Work out the finished part from the listing and answer in its coordinate system (mm). A direction names the side the tool comes from. Coordinates: 2 decimals unless noted, no trailing zeros. Order: outer loops, then holes, each group sorted by start corner. A loop starts at its lowest first (then second) coordinate and runs counter-clockwise, first axis right, second up. Notation, with made-up numbers: (69, 63.5) -> (105, 63.5) arc R5 cw to (105, 72.5) -> close; hole circle Ø10 at (59, 84.25). An arc over 180 degrees is marked (long way). Write item = value, one per line. Start each with the question number.
Q1. Straight lines are drawn through the part: L1, parallel to Z at x = 156, y = 10.5; L2, parallel to Z at x = 177, y = 2; L3, parallel to Y at x = 27.5, z = -49. For each, find the intervals that lie inside material, in ascending order. Write a range as from..to.
Q2. The part is cut by section B-B, the plane y = 13.5. Determine the outline of the cut face in (x, z), plus the area to 3 significant figures.
Q3. For a pull along X with two mould halves and no side action, classify faces 3 (the cylindrical face through (92.904, 1.521, -22.261)), 4 (the flat face through (-3, 0, -26)) as +X half, -X half, draft (parallel to the pull), parting line (faces both ways), or undercut.
Q4. The part is cut by section A-A, the plane x = -100. Determine the outline of the cut face in (y, z).
Q5. Flat-ended cylindrical pins translate along their axes: pin 1 (10.5 mm diameter, centred on x = 48.79, z = -48.79, fed in from +Y); pin 2 (4.5 mm diameter, centred on y = 10, z = -57, fed in from -X); pin 3 (0.9 mm diameter, centred on x = 175, y = 1, fed in from -Z). Find the tip coordinate at first contact, or state that the pin passes through.
Q6. Which of the six approach directions +Z, -Z, +X, -X, +Y, -Y give full straight-line access (tool end or side, diameter ignored) to faces 1 (the cylindrical face through (107.096, 1.521, 22.261)), 2 (the flat face through (2, 15, -57))?
Q7. The part is cut by section C-C, the plane x = 135. Determine the outline of the cut face in (y, z), plus the area to 3 significant figures.
```python
from build123d import *

# Parameters (mm, degrees)
SKETCH1_W                      = 370
SKETCH1_H                      = 114
SKETCH1_R                      = 4
SKETCH1_R_2                    = 24.5
BOSS_EXTRUDE1_DEPTH            = 3
EDGE_FLANGE1_STRIP_W           = 14
EDGE_FLANGE1_STRIP_H           = 3
EDGE_FLANGE1_STRIP_CUT_DEPTH   = 370
EDGE_FLANGE1_STRIP_2_W         = 14
EDGE_FLANGE1_STRIP_2_H         = 3
EDGE_FLANGE1_STRIP_CUT_2_DEPTH = 370
EDGE_FLANGE1_DEPTH             = 370
EDGE_FLANGE1_BEND_DEPTH        = 370
CUT_EXTRUDE1_REACH             = 198.087
SKETCH16_R                     = 3
SKETCH16_W                     = 25
SKETCH16_H                     = 58
CUT_EXTRUDE2_REACH             = 197.727
SKETCH17_R                     = 10.5
CUT_EXTRUDE3_START             = -185
CUT_EXTRUDE3_DEPTH             = 28
CUT_EXTRUDE3_START_2           = 157
CUT_EXTRUDE3_2_DEPTH           = 28


# Read off the part's stored shape, not the designer's step: Cut-Extrude3
# Sheet-metal steps are written as plain solids
with BuildPart() as part:
    # Sketch1 → Boss-Extrude1 (new body)
    with BuildSketch(Plane(origin=(0, 0, 0), x_dir=(1, 0, 0), z_dir=(0, 1, 0))):
        Rectangle(SKETCH1_W, SKETCH1_H)
        with Locations(Location((-48.790367902, 48.790367902, 0), (0, 0, 270))):
            Circle(SKETCH1_R, mode=Mode.SUBTRACT)
        with Locations(Location((48.790367902, 48.790367902, 0), (0, 0, 270))):
            Circle(SKETCH1_R, mode=Mode.SUBTRACT)
        with Locations(Location((48.790367902, -48.790367902, 0), (0, 0, 270))):
            Circle(SKETCH1_R, mode=Mode.SUBTRACT)
        with Locations(Location((-48.790367902, -48.790367902, 0), (0, 0, 270))):
            Circle(SKETCH1_R, mode=Mode.SUBTRACT)
        with Locations(Location((0, 0, 0), (0, 0, 270))):
            Circle(SKETCH1_R_2, mode=Mode.SUBTRACT)
    extrude(amount=BOSS_EXTRUDE1_DEPTH)

    # Edge-Flange1 strip (across the edge) → Edge-Flange1 strip cut (cut)
    with BuildSketch(Plane(origin=(-185, 3, 57), x_dir=(0, 0, -1), z_dir=(1, 0, 0))):
        with Locations((-6, -1.5)):
            Rectangle(EDGE_FLANGE1_STRIP_W, EDGE_FLANGE1_STRIP_H)
    extrude(amount=EDGE_FLANGE1_STRIP_CUT_DEPTH, mode=Mode.SUBTRACT)

    # Edge-Flange1 strip 2 (across the edge) → Edge-Flange1 strip cut 2 (cut)
    with BuildSketch(Plane(origin=(185, 3, -57), x_dir=(0, 0, 1), z_dir=(-1, 0, 0))):
        with Locations((-6, -1.5)):
            Rectangle(EDGE_FLANGE1_STRIP_2_W, EDGE_FLANGE1_STRIP_2_H)
    extrude(amount=EDGE_FLANGE1_STRIP_CUT_2_DEPTH, mode=Mode.SUBTRACT)

    # Edge-Flange1 section (across the edge) → Edge-Flange1 (add)
    with BuildSketch(Plane(origin=(-185, 3, 57), x_dir=(0, 0, -1), z_dir=(1, 0, 0))):
        with BuildLine():
            Line((-3, 1), (-3, 22))
            Line((-3, 22), (0, 22))
            Line((0, 22), (0, 1))
            ThreePointArc((0, 1), (0.292893219, 0.292893219), (1, 0))
            Line((1, 0), (1, -3))
            ThreePointArc((1, -3), (-1.828427125, -1.828427125), (-3, 1))
        make_face()
    extrude(amount=EDGE_FLANGE1_DEPTH)

    # Edge-Flange1 section 2 (across the edge) → Edge-Flange1 bend (add)
    with BuildSketch(Plane(origin=(185, 3, -57), x_dir=(0, 0, 1), z_dir=(-1, 0, 0))):
        with BuildLine():
            Line((-3, 1), (-3, 22))
            Line((-3, 22), (0, 22))
            Line((0, 22), (0, 1))
            ThreePointArc((0, 1), (0.292893219, 0.292893219), (1, 0))
            Line((1, 0), (1, -3))
            ThreePointArc((1, -3), (-1.828427125, -1.828427125), (-3, 1))
        make_face()
    extrude(amount=EDGE_FLANGE1_BEND_DEPTH)

    # Sketch16 → Cut-Extrude1 (cut, up to next)
    with BuildSketch(Plane.XZ, mode=Mode.PRIVATE) as cut_extrude1_sk1:
        with Locations(Location((177, 0, 0), (0, 0, 270))):
            Circle(SKETCH16_R)
    cut_extrude1_tool1 = extrude(cut_extrude1_sk1.sketch, amount=-CUT_EXTRUDE1_REACH, mode=Mode.PRIVATE) & part.part
    # Sketch16 → Cut-Extrude1 (cut, up to next)
    with BuildSketch(Plane.XZ, mode=Mode.PRIVATE) as cut_extrude1_sk2:
        with Locations(Location((145, 0, 0), (0, 0, 270))):
            Circle(SKETCH16_R)
    cut_extrude1_tool2 = extrude(cut_extrude1_sk2.sketch, amount=-CUT_EXTRUDE1_REACH, mode=Mode.PRIVATE) & part.part
    # Sketch16 → Cut-Extrude1 (cut, up to next)
    with BuildSketch(Plane.XZ, mode=Mode.PRIVATE) as cut_extrude1_sk3:
        with Locations((-172.5, 0)):
            Rectangle(SKETCH16_W, SKETCH16_H)
    cut_extrude1_tool3 = extrude(cut_extrude1_sk3.sketch, amount=-CUT_EXTRUDE1_REACH, mode=Mode.PRIVATE) & part.part
    add(cut_extrude1_tool1.solids().sort_by_distance((177, 0, 0))[0], mode=Mode.SUBTRACT)
    add(cut_extrude1_tool2.solids().sort_by_distance((145, 0, 0))[0], mode=Mode.SUBTRACT)
    add(cut_extrude1_tool3.solids().sort_by_distance((-172.5, 0, 0))[0], mode=Mode.SUBTRACT)

    # Sketch17 → Cut-Extrude2 (cut, up to next)
    with BuildSketch(Plane(origin=(0, 3, 0), x_dir=(1, 0, 0), z_dir=(0, 1, 0)), mode=Mode.PRIVATE) as cut_extrude2_sk1:
        with Locations(Location((-100, 30, 0), (0, 0, 270))):
            Circle(SKETCH17_R)
    cut_extrude2_tool1 = extrude(cut_extrude2_sk1.sketch, amount=-CUT_EXTRUDE2_REACH, mode=Mode.PRIVATE) & part.part
    # Sketch17 → Cut-Extrude2 (cut, up to next)
    with BuildSketch(Plane(origin=(0, 3, 0), x_dir=(1, 0, 0), z_dir=(0, 1, 0)), mode=Mode.PRIVATE) as cut_extrude2_sk2:
        with Locations(Location((100, 30, 0), (0, 0, 90))):
            Circle(SKETCH17_R)
    cut_extrude2_tool2 = extrude(cut_extrude2_sk2.sketch, amount=-CUT_EXTRUDE2_REACH, mode=Mode.PRIVATE) & part.part
    # Sketch17 → Cut-Extrude2 (cut, up to next)
    with BuildSketch(Plane(origin=(0, 3, 0), x_dir=(1, 0, 0), z_dir=(0, 1, 0)), mode=Mode.PRIVATE) as cut_extrude2_sk3:
        with Locations(Location((100, -30, 0), (0, 0, 270))):
            Circle(SKETCH17_R)
    cut_extrude2_tool3 = extrude(cut_extrude2_sk3.sketch, amount=-CUT_EXTRUDE2_REACH, mode=Mode.PRIVATE) & part.part
    # Sketch17 → Cut-Extrude2 (cut, up to next)
    with BuildSketch(Plane(origin=(0, 3, 0), x_dir=(1, 0, 0), z_dir=(0, 1, 0)), mode=Mode.PRIVATE) as cut_extrude2_sk4:
        with Locations(Location((-100, -30, 0), (0, 0, 90))):
            Circle(SKETCH17_R)
    cut_extrude2_tool4 = extrude(cut_extrude2_sk4.sketch, amount=-CUT_EXTRUDE2_REACH, mode=Mode.PRIVATE) & part.part
    add(cut_extrude2_tool1.solids().sort_by_distance((-100, 3, -30))[0], mode=Mode.SUBTRACT)
    add(cut_extrude2_tool2.solids().sort_by_distance((100, 3, -30))[0], mode=Mode.SUBTRACT)
    add(cut_extrude2_tool3.solids().sort_by_distance((100, 3, 30))[0], mode=Mode.SUBTRACT)
    add(cut_extrude2_tool4.solids().sort_by_distance((-100, 3, 30))[0], mode=Mode.SUBTRACT)

    # Cut-Extrude3 outline → Cut-Extrude3 (cut)
    with BuildSketch(Plane.YZ.offset(CUT_EXTRUDE3_START)):
        with BuildLine():
            ThreePointArc((4, -57), (3.292893219, -56.707106781), (3, -56))
            Line((3, -56), (0, -56))
            ThreePointArc((0, -56), (1.171572875, -58.828427125), (4, -60))
            Line((4, -60), (25, -60))
            Line((25, -60), (25, -57))
            Line((25, -57), (4, -57))
        make_face()
        with BuildLine():
            ThreePointArc((4, 60), (1.171572875, 58.828427125), (0, 56))
            Line((0, 56), (3, 56))
            ThreePointArc((3, 56), (3.292893219, 56.707106781), (4, 57))
            Line((4, 57), (25, 57))
            Line((25, 57), (25, 60))
            Line((25, 60), (4, 60))
        make_face()
    extrude(amount=CUT_EXTRUDE3_DEPTH, mode=Mode.SUBTRACT)

    # Cut-Extrude3 2 outline → Cut-Extrude3 2 (cut)
    with BuildSketch(Plane.YZ.offset(CUT_EXTRUDE3_START_2)):
        with BuildLine():
            ThreePointArc((4, -57), (3.292893219, -56.707106781), (3, -56))
            Line((3, -56), (0, -56))
            ThreePointArc((0, -56), (1.171572875, -58.828427125), (4, -60))
            Line((4, -60), (25, -60))
            Line((25, -60), (25, -57))
            Line((25, -57), (4, -57))
        make_face()
        with BuildLine():
            ThreePointArc((4, 60), (1.171572875, 58.828427125), (0, 56))
            Line((0, 56), (3, 56))
            ThreePointArc((3, 56), (3.292893219, 56.707106781), (4, 57))
            Line((4, 57), (25, 57))
            Line((25, 57), (25, 60))
            Line((25, 60), (4, 60))
        make_face()
    extrude(amount=CUT_EXTRUDE3_2_DEPTH, mode=Mode.SUBTRACT)


solid = part.part
```
Model answer:
q1.L1 = -60..-57, 57..60
q1.L2 = -56..-3, 3..56
q1.L3 = 0..3
q2.outline = (-157, -60) -> (157, -60) -> (157, -57) -> (-157, -57) -> close; (-157, 57) -> (157, 57) -> (157, 60) -> (-157, 60) -> close
q2.area = 1,880 mm2
q3.face_3 = undercut
q3.face_4 = draft
q4.outline = (0, -56) arc R4 ccw to (4, -60) -> (25, -60) -> (25, -57) -> (4, -57) arc R1 cw to (3, -56) -> (3, -40.5) -> (0, -40.5) -> close; (0, -19.5) -> (3, -19.5) -> (3, 19.5) -> (0, 19.5) -> close; (0, 40.5) -> (3, 40.5) -> (3, 56) arc R1 cw to (4, 57) -> (25, 57) -> (25, 60) -> (4, 60) arc R4 ccw to (0, 56) -> close
q5.pin_1 = 3
q5.pin_2 = -157
q5.pin_3 = -56
q6.face_1 = +Y, -Y
q6.face_2 = +X, -X, +Y
q7.outline = (0, -56) arc R4 ccw to (4, -60) -> (25, -60) -> (25, -57) -> (4, -57) arc R1 cw to (3, -56) -> (3, 56) arc R1 cw to (4, 57) -> (25, 57) -> (25, 60) -> (4, 60) arc R4 ccw to (0, 56) -> close
q7.area = 486 mm2
